from build123d import *

# Parameters (mm, degrees)
SKETCH1_W           = 28
SKETCH1_H           = 28
SKETCH1_W_2         = 24
SKETCH1_H_2         = 24
BOSS_EXTRUDE1_DEPTH = 15
SKETCH2_W           = 28
SKETCH2_H           = 28
BOSS_EXTRUDE2_DEPTH = 2
CUT_EXTRUDE1_REACH  = 19
SKETCH3_R           = 4.25


with BuildPart() as part:
    # Sketch1 → Boss-Extrude1 (new body)
    with BuildSketch(Plane(origin=(0, 0, 0), x_dir=(1, 0, 0), z_dir=(0, 1, 0))):
        Rectangle(SKETCH1_W, SKETCH1_H)
        Rectangle(SKETCH1_W_2, SKETCH1_H_2, mode=Mode.SUBTRACT)
    extrude(amount=BOSS_EXTRUDE1_DEPTH)

    # Sketch2 → Boss-Extrude2 (add)
    with BuildSketch(Plane(origin=(0, 15, 0), x_dir=(1, 0, 0), z_dir=(0, 1, 0))):
        Rectangle(SKETCH2_W, SKETCH2_H)
    extrude(amount=BOSS_EXTRUDE2_DEPTH)

    # Sketch3 → Cut-Extrude1 (cut, up to next)
    with BuildSketch(Plane(origin=(0, 17, 0), x_dir=(1, 0, 0), z_dir=(0, 1, 0)), mode=Mode.PRIVATE) as cut_extrude1_sk1:
        Circle(SKETCH3_R)
    cut_extrude1_tool1 = extrude(cut_extrude1_sk1.sketch, amount=-CUT_EXTRUDE1_REACH, mode=Mode.PRIVATE) & part.part
    add(cut_extrude1_tool1.solids().sort_by_distance((0, 17, 0))[0], mode=Mode.SUBTRACT)


solid = part.part
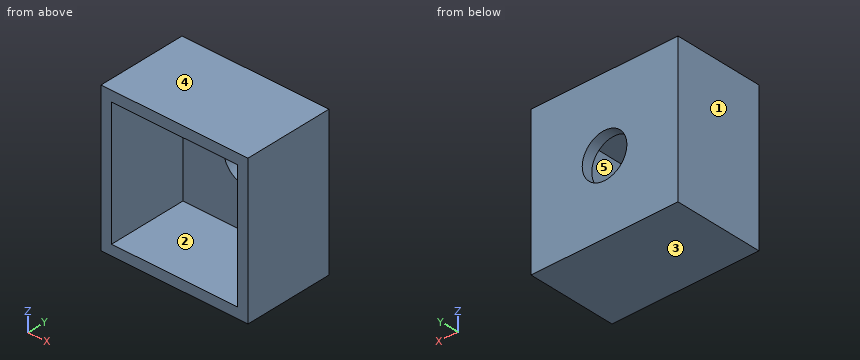
Here's how the part is built. I have some questions about the finished solid (model axes, mm). Face numbers are marked on the shaded views. A direction names the side the tool comes from. Coordinates: 2 decimals unless noted, no trailing zeros. Write each loop counter-clockwise with the first axis right and the second up, starting at its lowest first coordinate (ties: lowest second). Pieces come first, ordered by that corner, then holes.
1) I'm going to push a flat-ended pin straight in: pin 1 (11 mm diameter, centred on x = 0, z = 0, fed in from -Y). Where does the tip first touch, or does it pass through?
Filled in:
pin 1: stops at y = 15
2) If we section it at D-D (z = 7): List the corners of the cut face in (x, y) for me.
Filled in:
outline: (-14, 0) - (-12, 0) - (-12, 15) - (12, 15) - (12, 0) - (14, 0) - (14, 17) - (-14, 17) - close
3) Thinking about a two-plate mould opening in Z: for the marked faces 1, 2 and 3, which applies, +Z half, -Z half, draft (parallel to the pull), parting line (faces both ways), or undercut?
Filled in:
face 1: draft
face 2: undercut
face 3: -Z half
4) If we section it at C-C (y = 12.25): List the corners of the cut face in (x, z) for me.
Filled in:
outline: (-14, -14) - (14, -14) - (14, 14) - (-14, 14) - close; hole (-12, -12) - (12, -12) - (12, 12) - (-12, 12) - close
5) If I drill on line 1 (X direction, y = 10.5, z = -7); line 2 (X direction, y = 15.8, z = 0), over which ranges is the centre line in solid material (lowest first)?
Filled in:
line 1: x = -14 to -12, 12 to 14
line 2: x = -14 to -4.25, 4.25 to 14
6) If we section it at B-B (x = 0): List the corners of the cut face in (y, z) for me.
Filled in:
outline: (0, -14) - (17, -14) - (17, -4.25) - (15, -4.25) - (15, -12) - (0, -12) - close; (0, 12) - (15, 12) - (15, 4.25) - (17, 4.25) - (17, 14) - (0, 14) - close
7) If we section it at A-A (z = 0): List the corners of the cut face in (x, y) for me.
Filled in:
outline: (-14, 0) - (-12, 0) - (-12, 15) - (-4.25, 15) - (-4.25, 17) - (-14, 17) - close; (4.25, 15) - (12, 15) - (12, 0) - (14, 0) - (14, 17) - (4.25, 17) - close
8) Which directions (+Z, -Z, +X, -X, +Y, -Y) give clear straight access to the entire face, cutting with the end or side of a thin tool? Please do the marked faces 4 and 5.
Filled in:
face 4: +Z, +X, -X, +Y, -Y
face 5: -Y
